Check sheet for the modelled part. Datum: model origin and axes. Units: mm. A direction names the side the tool comes from. Round coordinates to 2 decimals unless told otherwise and drop trailing zeros. Loops run counter-clockwise (first coordinate to the right, second up) from the corner with the lowest first, then second, coordinate; pieces in that order, holes last. Notation, with made-up numbers: (-11, 36) - (36, 36) arc R13 cw to (36, 60) - close; hole circle Ø2 at (31.25, -40). An arc over 180 degrees is marked (long way). Answer in a Markdown table with one row per item. Add a question column.
(1) Mould release check, pull along Y, two halves, no side actions. Record for faces 3 (the cylindrical face through (58.748, 6.901, -0.493)), 4 (the flat face through (-1, -21, 3)), 5 (the cylindrical face through (-58.748, 7.099, -0.493)), 6 (the flat face through (-85.5, -5.6, -0.5)): +Y half, -Y half, draft (parallel to the pull), parting line (faces both ways), or undercut.
(2) Thickness scan on line 1 along Y through (x, z) = (-34, 3.6); line 2 along Z through (x, y) = (64, 5); line 3 along Y through (x, z) = (-56.5, -0.65). Record the ranges inside material, lowest first.
(3) Cross-section at C-C on x = 24.5. Enter the section's corners in (y, z).
(4) Gauge pin test, flat ends, axial feed: pin 1 (10 mm diameter, centred on x = 5.5, y = -2, fed in from +Z); pin 2 (3.5 mm diameter, centred on x = 16.5, z = 2.5, fed in from +Y). Record the tip position at first contact, or that the pin passes through.
(5) Cross-section at A-A on x = -56.5. Enter the section's corners in (y, z), then the cut area to 3 significant figures.
(6) Cross-section at D-D on z = 2. Enter the section's corners in (x, y), then the cut area to 3 significant figures.
(7) Access from +Z, -Z, +X, -X, +Y, -Y to the whole of each face (thin tool, end or side, straight path). Record for faces 1 (the flat face through (-1, -2, -1)), 2 (the flat face through (-1, -2, 0)).
(8) Cross-section at B-B on y = 7. Enter the section's corners in (x, z).
from build123d import *

# Parameters (mm, degrees)
ESQUISSE1_W                           = 171
ESQUISSE1_H                           = 34
ESQUISSE1_R                           = 2.25
T_LE_DE_BASE_PLI_E1_DEPTH             = 1
T_LE_PLI_E_SUR_AR_TE1_STRIP_W         = 5.4732
T_LE_PLI_E_SUR_AR_TE1_STRIP_H         = 1
T_LE_PLI_E_SUR_AR_TE1_STRIP_CUT_DEPTH = 171
T_LE_PLI_E_SUR_AR_TE1_DEPTH           = 171
CONG_1_R                              = 2


# Sheet-metal steps are written as plain solids
with BuildPart() as part:
    # Esquisse1 → Tôle de base pliée1 (new body)
    with BuildSketch(Plane.XY):
        with Locations((0, -3)):
            Rectangle(ESQUISSE1_W, ESQUISSE1_H)
        with Locations((-56.5, 7)):
            Circle(ESQUISSE1_R, mode=Mode.SUBTRACT)
        with Locations(Location((56.5, 7, 0), (0, 0, 180))):
            Circle(ESQUISSE1_R, mode=Mode.SUBTRACT)
    extrude(amount=-T_LE_DE_BASE_PLI_E1_DEPTH)

    # Tôle pliée sur arête1 strip (across the edge) → Tôle pliée sur arête1 strip cut (cut)
    with BuildSketch(Plane(origin=(-85.5, -20, 0), x_dir=(0, 1, 0), z_dir=(1, 0, 0))):
        with Locations((-2, -0.5)):
            Rectangle(T_LE_PLI_E_SUR_AR_TE1_STRIP_W, T_LE_PLI_E_SUR_AR_TE1_STRIP_H)
    extrude(amount=T_LE_PLI_E_SUR_AR_TE1_STRIP_CUT_DEPTH, mode=Mode.SUBTRACT)

    # Tôle pliée sur arête1 section (across the edge) → Tôle pliée sur arête1 (add)
    with BuildSketch(Plane(origin=(-85.5, -20, 0), x_dir=(0, 1, 0), z_dir=(1, 0, 0))):
        with BuildLine():
            Line((-1, 0.7366), (-1, 5))
            Line((-1, 5), (0, 5))
            Line((0, 5), (0, 0.7366))
            ThreePointArc((0, 0.7366), (0.215745145, 0.215745145), (0.7366, 0))
            Line((0.7366, 0), (0.7366, -1))
            ThreePointArc((0.7366, -1), (-0.491361636, -0.491361636), (-1, 0.7366))
        make_face()
    extrude(amount=T_LE_PLI_E_SUR_AR_TE1_DEPTH)

    # Congé1
    cong_1_edges = [part.edges().sort_by_distance(p)[0] for p in [
        (-85.5, -20.5, 5),
        (85.5, -20.5, 5),
        (-85.5, 14, -0.5),
        (85.5, 14, -0.5),
    ]]
    fillet(cong_1_edges, radius=CONG_1_R)


solid = part.part
Answers:
| question | item | result |
|---|---|---|
| 1 | face 3 | undercut |
| 1 | face 4 | -Y half |
| 1 | face 5 | undercut |
| 1 | face 6 | draft |
| 2 | line 1 | y = -21 to -20 |
| 2 | line 2 | z = -1 to 0 |
| 2 | line 3 | y = -20.31 to 4.75, 9.25 to 14 |
| 3 | outline | (-21, 0.74) arc R1.74 ccw to (-19.26, -1) - (14, -1) - (14, 0) - (-19.26, 0) arc R0.74 cw to (-20, 0.74) - (-20, 5) - (-21, 5) - close |
| 4 | pin 1 | stops at z = 0 |
| 4 | pin 2 | stops at y = -20 |
| 5 | outline | (-21, 0.74) arc R1.74 ccw to (-19.26, -1) - (4.75, -1) - (4.75, 0) - (-19.26, 0) arc R0.74 cw to (-20, 0.74) - (-20, 5) - (-21, 5) - close; (9.25, -1) - (14, -1) - (14, 0) - (9.25, 0) - close |
| 5 | area | 35.0 mm^2 |
| 6 | outline | (-85.5, -21) - (85.5, -21) - (85.5, -20) - (-85.5, -20) - close |
| 6 | area | 171 mm^2 |
| 7 | face 1 | -Z, +X, -X, +Y, -Y |
| 7 | face 2 | +Z, +X, -X, +Y |
| 8 | outline | (-85.5, -1) - (-58.75, -1) - (-58.75, 0) - (-85.5, 0) - close; (-54.25, -1) - (54.25, -1) - (54.25, 0) - (-54.25, 0) - close; (58.75, -1) - (85.5, -1) - (85.5, 0) - (58.75, 0) - close |
